Part model, mm, in its own coordinate system. Face numbers are marked on the shaded views. A direction names the side the tool comes from. Give positions to 0.01 mm unless a question says otherwise; leave off trailing zeros. Order: outer loops, then holes, each group sorted by start corner. A loop starts at its lowest first (then second) coordinate and runs counter-clockwise, first axis right, second up. Notation, with made-up numbers: M 38,-21.5 L 72,-21.5 A32 cw 72,5.5 Z; hole C 1,-10 d8. An arc over 180 degrees is marked long. Return JSON: item names as keys, results as strings.
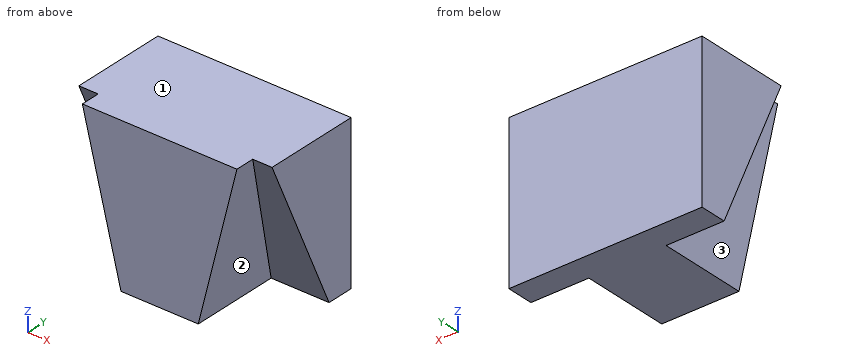
Solid Edge part; units mm, degrees
sketch "Sketch1" plane through (0, 0, 0) normal (0, -1, 0) x (1, 0, 0)
  line L0 (20, 20) -> (10, -20)
  line L1 (-10, -20) -> (10, -20)
  line L2 (-10, -20) -> (-20, 20)
  line L3 (20, 20) -> (-20, 20)
extrude "Protrusion1" add sketch "Sketch1" against normal blind 30
sketch "Sketch2" plane through (0, 0, 0) normal (1, 0, 0) x (0, 1, 0)
  line L0 (30, -20) -> (23.0281, -20)
  line L1 (5, 20) -> (23.0281, -20)
  line L2 (30, 20) -> (5, 20)
  line L3 (30, -13.924) -> (30, 20)
extrude "ExtrudedProtrusion_3" add sketch "Sketch2" along normal blind 25 material side at (0, 26.514, -19.95)
sketch "Sketch3" plane through (0, 0, 0) normal (1, 0, 0) x (0, 1, 0)
  line L0 (30, -20) -> (23.0281, -20)
  line L1 (5, 20) -> (23.0281, -20)
  line L2 (30, 20) -> (5, 20)
  line L3 (30, -13.924) -> (30, 20)
extrude "ExtrudedProtrusion_4" add sketch "Sketch3" against normal blind 25 material side at (0, 26.514, -19.95)
Q1. 3-axis set-ups, long thin cutter, end or side, ignore diameter. For the marked faces 1, 2 and 3: which of +Z, -Z, +X, -X, +Y, -Y reach the whole face in a straight line?
Established:
{"face 1": "+Z, +X, -X, +Y, -Y", "face 2": "-Z, +X, -Y", "face 3": "-Z, -X, -Y"}
Q2. Probe line 1 along Y through (x, z) = (22.5, -6.5); line 2 along Y through (x, z) = (-18.5, 5); line 3 along X through (y, z) = (6, 4). List the from-to ranges inside material, lowest first.
Established:
{"line 1": "y = 16.94 to 30", "line 2": "y = 11.76 to 30", "line 3": "x = -16 to 16"}
Q3. Band-saw the part on A-A (z = -5). Give the cut face in (x, y), then the cut area to 3 significant figures.
Established:
{"outline": "M -25,16.27 L -13.75,16.27 L -13.75,0 L 13.75,0 L 13.75,16.27 L 25,16.27 L 25,30 L -25,30 Z", "area": "1,130 mm²"}
Q4. Band-saw the part on C-C (x = 18). Give the cut face in (y, z), then the cut area to 3 significant figures.
Established:
{"outline": "M 0,12 L 8.61,12 L 23.03,-20 L 30,-20 L 30,20 L 0,20 Z", "area": "694 mm²"}
Q5. Band-saw the part on D-D (y = 4). Give the cut face in (x, z).
Established:
{"outline": "M -20,20 L -10,-20 L 10,-20 L 20,20 Z"}
Q6. Band-saw the part on B-B (y = 8.5). Give the cut face in (x, z).
Established:
{"outline": "M -25,12.23 L -18.06,12.23 L -10,-20 L 10,-20 L 18.06,12.23 L 25,12.23 L 25,20 L -25,20 Z"}
Q7. Pin check, flat tip, straight feed: pin 1 (10 mm diameter, centred on y = 11, z = 3, fed in from +X). Stop position of the tip, or through.
Established:
{"pin 1": "stops at x = 25"}
